```python
from build123d import *

# Parameters (mm, degrees)
F0_R     = 18.5
F0_R_2   = 14.75
F1_DEPTH = 3.25
F3_DEPTH = 25
F4_R     = 1


with BuildPart() as f1:
    # F0 (on Top) → F1 (new body)
    with BuildSketch(Plane.XY):
        Circle(F0_R)
        Circle(F0_R_2, mode=Mode.SUBTRACT)
    extrude(amount=F1_DEPTH)

    # F2 (on face) → F3 (cut)
    with BuildSketch(Plane.XY.offset(3.25)):
        with BuildLine():
            Line((14, 9.5), (15.874508, 9.5))
            ThreePointArc((15.874508, 9.5), (14.993431, 10.837298), (14, 12.093387))
            Line((14, 12.093387), (14, 9.5))
        make_face()
    extrude(amount=-F3_DEPTH, mode=Mode.SUBTRACT)

    # F4
    f4_edges = [f1.edges().sort_by_distance(p)[0] for p in [
        (-14.993431, -10.837298, 3.25),
    ]]
    fillet(f4_edges, radius=F4_R)


solid = f1.part
```
Work out the finished part from the listing and answer in its coordinate system (mm). A direction names the side the tool comes from. Give positions to 0.01 mm unless a question says otherwise; leave off trailing zeros. Loops run counter-clockwise (first coordinate to the right, second up) from the corner with the lowest first, then second, coordinate; pieces in that order, holes last. Notation, with made-up numbers: (28, -13) -> (66, -13) arc R16 ccw to (66, -4) -> close; hole circle Ø6 at (78, -22.5). An arc over 180 degrees is marked (long way). Write item = value, one per line. Start each with the question number.
(1) Which of the six approach directions +Z, -Z, +X, -X, +Y, -Y give full straight-line access (tool end or side, diameter ignored) to faces 4 (the cylindrical face through (-15.44, -10.19, 1.11)), 5 (the flat face through (14, 11, 2))?
(2) Find section A-A on y = 0. Give the vertices of the cut face in (x, z), and give its area (3 significant figures).
(3) Find section C-C on z = 1.2. Give the vertices of the cut face in (x, y).
(4) Find the intervals of material crossed by probe 1 along Y at (x, z) = (0, 1.7); probe 2 along Y at (x, z) = (-7.5, 1.75); probe 3 along X at (y, z) = (-9.5, 3), in increasing order. Write a range as from..to.
(5) Given pin 1 Ø0.6 at (x, z) = (14.5, 2) entering from +Y; pin 2 Ø1.5 at (x, y) = (-4.5, -12) entering from -Z; pin 3 Ø1.5 at (x, y) = (-13, 8) entering from -Z, each flat-ended and moving along its own axis, determine where each tip first touches the part or whether it passes through.
(6) The mould has two halves that part along Y. Classify faces 1 (the flat face through (15, 9.5, 2)), 2 (the flat face through (-6, 14, 0)), 3 (the cylindrical face through (14.07, 4.43, 1.6)): +Y half, -Y half, draft (parallel to the pull), parting line (faces both ways), or undercut.
From the geometry:
q1.face_4 = +Z, -Z
q1.face_5 = +Z, -Z, +X, +Y
q2.outline = (-18.5, 0) -> (-14.75, 0) -> (-14.75, 3.25) -> (-17.5, 3.25) arc R1 ccw to (-18.5, 2.25) -> close; (14.75, 0) -> (18.5, 0) -> (18.5, 2.25) arc R1 ccw to (17.5, 3.25) -> (14.75, 3.25) -> close
q2.area = 23.9 mm^2
q3.outline = (14, 9.5) -> (14, 12.09) arc R18.5 ccw (long way) to (15.87, 9.5) -> close; hole circle Ø29.5 at (0, 0)
q4.probe_1 = -18.5..-14.75, 14.75..18.5
q4.probe_2 = -16.91..-12.7, 12.7..16.91
q4.probe_3 = -15.48..-11.28, 11.28..15.48
q5.pin_1 = 9.5
q5.pin_2 = through
q5.pin_3 = 0
q6.face_1 = +Y half
q6.face_2 = draft
q6.face_3 = undercut
